CAD build for the part. Positions are in the model's coordinates, mm. A direction names the side the tool comes from. Round coordinates to 2 decimals unless told otherwise and drop trailing zeros. Loops run counter-clockwise (first coordinate to the right, second up) from the corner with the lowest first, then second, coordinate; pieces in that order, holes last. Notation, with made-up numbers: M 43,13.25 L 52,13.25 A25 ccw 52,33.25 Z; hole C 53,73.5 d8. An arc over 180 degrees is marked long. Put each result on its own line as item: value. Start each with the question number.
from build123d import *

# Parameters (mm, degrees)
F0_R     = 2.7559
F1_DEPTH = 19.05
F2_DEPTH = 12.7
F3_DEPTH = 25.4
F4_R     = 4.7625
F5_DEPTH = 19.051
F6_R     = 4.7625
F7_DEPTH = 7.9375


with BuildPart() as f1:
    # F0 (on Top) → F1 (new body)
    with BuildSketch(Plane.XY):
        with BuildLine():
            Line((-55.9988788353, 44.7037652499), (-76.5532134465, 44.4946135236))
            ThreePointArc((-76.5532134465, 44.4946135236), (-126.7555499575, -5.2172696713), (-78.5805513553, -56.8962347501))
            Line((-78.5805513553, -56.8962347501), (-55.9988788353, -56.8962347501))
            Line((-55.9988788353, -56.8962347501), (-55.9988788353, 44.7037652499))
        make_face()
        with Locations((-106.7988788353, -23.8762347501)):
            Circle(F0_R, mode=Mode.SUBTRACT)
        with Locations((-106.7988788353, 11.4746135236)):
            Circle(F0_R, mode=Mode.SUBTRACT)
    extrude(amount=F1_DEPTH)

    # F2 (add): a face of the model
    f2_faces = [f1.faces().sort_by_distance(p)[0] for p in [
        (-55.9988788353, -6.0962347501, 9.525),
    ]]
    extrude(f2_faces, amount=F2_DEPTH)

    # F3 (add): a face of the model
    f3_faces = [f1.faces().sort_by_distance(p)[0] for p in [
        (-43.2988788353, -6.0962347501, 9.525),
    ]]
    extrude(f3_faces, amount=F3_DEPTH)

    # F4 (on face) → F5 (cut, through all)
    with BuildSketch(Plane.XY.offset(19.05)):
        with Locations((-68.6988788353, -6.0962347501)):
            Circle(F4_R)
    extrude(amount=-F5_DEPTH, mode=Mode.SUBTRACT)

    # F6 (on face) → F7 (cut)
    with BuildSketch(Plane(origin=(0, 0, 0), x_dir=(1, 0, 0), z_dir=(0, 0, -1))):
        Polygon((-75.8616788353, 3.1293058456), (-71.6658077398, -1.0665652499), (-65.7102826454, -1.0665652499), (-61.5360788353, 3.1076385602), (-61.5360788353, 9.0631636547), (-65.7319499307, 13.2590347501), (-71.6658077398, 13.2590347501), (-75.8616788353, 9.0631636547), align=None)
        with Locations((-68.6988788353, 6.0962347501)):
            Circle(F6_R, mode=Mode.SUBTRACT)
    extrude(amount=-F7_DEPTH, mode=Mode.SUBTRACT)


solid = f1.part
(1) Mould opens along X. For faces 3 (the cylindrical face through (-126.72, -4.12, 9.39)), 4 (the flat face through (-37, 44.704, 9)), 5 (the flat face through (-63.652, -0.991, 3.913)) say: +X half, -X half, draft (parallel to the pull), parting line (faces both ways), or undercut.
(2) Cut at C-C on y = 22.5. List the corners of the cut face in (x, z), and give its area (3 significant figures).
(3) Cut at A-A on x = -68.5. List the corners of the cut face in (y, z).
(4) Cut at D-D on z = 6. List the corners of the cut face in (x, y).
(5) Drill centre lines: line 1 along X through (y, z) = (-6, 10); line 2 along X through (y, z) = (12.5, 17.25); line 3 along Z through (x, y) = (-70.5, -0.5). Where is each one in solid material? Low to high.
(6) Tool access for faces 1 (the flat face through (-61, -7, 19.05)), 2 (the flat face through (-69, -13.259, 4)): list every direction of +Z, -Z, +X, -X, +Y, -Y with a clear straight run to the whole face (end or side of a thin tool).
(7) Flat gauge pins, fed straight in: pin 1 Ø1 at (x, y) = (-86.5, 18.5) entering from -Z; pin 2 Ø1.5 at (x, z) = (-109.5, 4.5) entering from +Y; pin 3 Ø4.5 at (x, z) = (-70, 2.5) entering from +Y; pin 4 Ø3.5 at (x, y) = (-106.8, 11.47) entering from +Z. Where does each tip first touch, or does it go through?
Taken from the geometry:
1. face 3: -X half
1. face 4: draft
1. face 5: undercut
2. outline: M -117.84,0 L -17.9,0 L -17.9,19.05 L -117.84,19.05 Z
2. area: 1,900 mm2
3. outline: M -56.9,0 L -13.26,0 L -13.26,7.94 L -10.85,7.94 L -10.85,19.05 L -56.9,19.05 Z; M -1.34,7.94 L 1.07,7.94 L 1.07,0 L 44.58,0 L 44.58,19.05 L -1.34,19.05 Z
4. outline: M -78.58,-56.9 L -17.9,-56.9 L -17.9,44.7 L -56,44.7 L -76.55,44.49 A50.73 ccw Z; hole C -106.8,-23.88 d5.51; hole C -106.8,11.47 d5.51; hole M -75.86,-9.06 L -71.67,-13.26 L -65.73,-13.26 L -61.54,-9.06 L -61.54,-3.11 L -65.71,1.07 L -71.67,1.07 L -75.86,-3.13 Z
5. line 1: -126.77 to -73.46, -63.94 to -17.9
5. line 2: -123.18 to -109.36, -104.24 to -17.9
5. line 3: 7.94 to 19.05
6. face 1: +Z, +X, -X, +Y, -Y
6. face 2: -Z
7. pin 1: z = 0
7. pin 2: y = 32.54
7. pin 3: y = 44.58
7. pin 4: through
